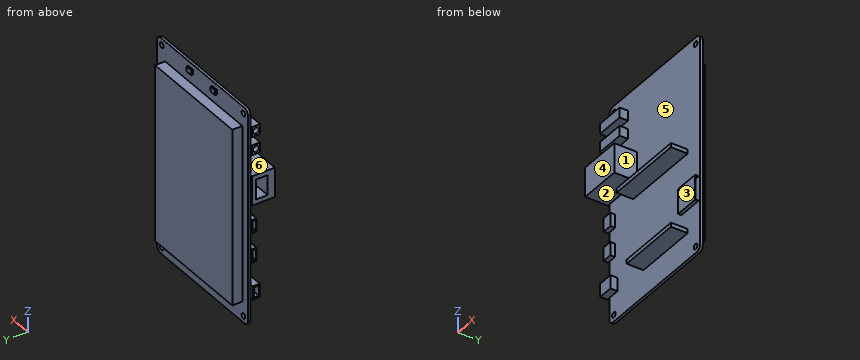
Autodesk Inventor part; units mm, degrees
ref_plane "YZ Plane" through (0, 0, 0) normal (1, 0, 0) x (0, 1, 0)
ref_plane "XZ Plane" through (0, 0, 0) normal (0, 1, 0) x (-1, 0, 0)
ref_plane "XY Plane" through (0, 0, 0) normal (0, 0, 1) x (1, 0, 0)
sketch "Esquisse1" plane through (0, 0, 0) normal (0, 1, 0) x (-1, 0, 0)
  line L0 (40, 65) -> (-40, 65)
  line L1 (-40, 65) -> (-40, -65)
  line L2 (-40, -65) -> (40, -65)
  line L3 (40, -65) -> (40, 65)
  point P0 (0, 0)
  dimension "d0" = 130
  dimension "d1" = 80
  dimension "d2" = 40
  dimension "d3" = 65
extrude "Extrusion1" add sketch "Esquisse1" along normal blind 1.6
sketch "Esquisse2" plane through (0, 1.6, 0) normal (0, 1, 0) x (1, 0, 0)
  circle A0 centre (-36, -61) radius 1.6
  circle A1 centre (-36, 61) radius 1.6
  circle A2 centre (36, 61) radius 1.6
  circle A3 centre (36, -61) radius 1.6
  point P0 (0, 0)
  dimension "d6" = 3.2
  dimension "d7" = 3.2
  dimension "d8" = 3.2
  dimension "d9" = 3.2
  dimension "d10" = 122
  dimension "d11" = 122
  dimension "d12" = 72
  dimension "d13" = 72
  dimension "d14" = 61
  dimension "d15" = 36
  dimension "d16" = 36
  dimension "d17" = 61
extrude "Extrusion2" cut sketch "Esquisse2" against normal blind 1.6
fillet "Congé1" radius 3.2 4 edges at (-40, 0.8, 65) (40, 0.8, 65) (40, 0.8, -65) (-40, 0.8, -65)
sketch "Esquisse3" plane through (0, 1.6, 0) normal (0, 1, 0) x (1, 0, 0)
  line L0 (-35, -53) -> (33, -53)
  line L1 (33, -53) -> (33, 53)
  line L2 (33, 53) -> (-35, 53)
  line L3 (-35, 53) -> (-35, -53)
  line L4 (40, -61.8) -> (40, 61.8)
  line L5 (36.8, 65) -> (-36.8, 65)
  point P0 (0, 0)
  dimension "d21" = 106
  dimension "d22" = 68
  dimension "d23" = 7
  dimension "d24" = 12
extrude "Extrusion3" add sketch "Esquisse3" along normal blind 6
sketch "Esquisse4" plane through (0, 1.6, 0) normal (0, 1, 0) x (1, 0, 0)
  line L0 (-12.5, -59) -> (-8.5, -59)
  line L1 (-8.5, -59) -> (-8.5, -62)
  line L2 (-8.5, -62) -> (-12.5, -62)
  line L3 (-12.5, -62) -> (-12.5, -59)
  line L4 (8.5, -59) -> (12.5, -59)
  line L5 (12.5, -59) -> (12.5, -62)
  line L6 (12.5, -62) -> (8.5, -62)
  line L7 (8.5, -62) -> (8.5, -59)
  line L8 (-36.8, -65) -> (36.8, -65)
  line L9 (40, -61.8) -> (40, 61.8)
  point P0 (0, 0)
  dimension "d27" = 4
  dimension "d28" = 3
  dimension "d29" = 6
  dimension "d30" = 6
  dimension "d31" = 4
  dimension "d32" = 17
  dimension "d33" = 27.5
extrude "Extrusion4" add sketch "Esquisse4" along normal blind 1
sketch "Esquisse5" plane through (0, 0, 0) normal (0, -1, 0) x (1, 0, 0)
  line L0 (-41.9, -48.5) -> (-32.9, -48.5)
  line L1 (-32.9, -48.5) -> (-32.9, -40.5)
  line L2 (-32.9, -40.5) -> (-41.9, -40.5)
  line L3 (-41.9, -40.5) -> (-41.9, -48.5)
  line L4 (36.8, -65) -> (-36.8, -65)
  line L5 (-40, -61.8) -> (-40, 61.8)
  point P0 (0, 0)
  dimension "d36" = 8
  dimension "d37" = 9
  dimension "d38" = 16.5
  dimension "d39" = 1.9
extrude "Extrusion5" add sketch "Esquisse5" along normal blind 4.2
sketch "Esquisse6" plane through (0, 0, 0) normal (0, -1, 0) x (1, 0, 0)
  line L0 (-35, 53) -> (-35, -53)
  line L1 (-41, -26.7) -> (-35, -26.7)
  line L2 (-35, -26.7) -> (-35, -18.7)
  line L3 (-35, -18.7) -> (-41, -18.7)
  line L4 (-41, -18.7) -> (-41, -26.7)
  line L5 (-41, -9.1) -> (-35, -9.1)
  line L6 (-35, -9.1) -> (-35, -1.1)
  line L7 (-35, -1.1) -> (-41, -1.1)
  line L8 (-41, -1.1) -> (-41, -9.1)
  line L9 (-32.9, -40.5) -> (-41.9, -40.5)
  line L10 (-40, -61.8) -> (-40, 61.8)
  point P0 (0, 0)
  dimension "d42" = 8
  dimension "d43" = 8
  dimension "d44" = 6
  dimension "d45" = 13.8
  dimension "d46" = 9.6
  dimension "d47" = 1
extrude "Extrusion6" add sketch "Esquisse6" along normal blind 2.8 contours L0 L5 L10 L7 | L10 L5 L8 L7 | L0 L1 L10 L3 | L10 L1 L4 L3
sketch "Esquisse7" plane through (0, 0, 0) normal (0, -1, 0) x (1, 0, 0)
  line L0 (-41.4, 7.9) -> (-15.7, 7.9)
  line L1 (-15.7, 7.9) -> (-15.7, 25.6)
  line L2 (-15.7, 25.6) -> (-41.4, 25.6)
  line L3 (-41.4, 25.6) -> (-41.4, 7.9)
  line L4 (-35, -1.1) -> (-41, -1.1)
  line L5 (-40, -1.1) -> (-40, 61.8)
  point P0 (0, 0)
  dimension "d50" = 25.7
  dimension "d51" = 17.7
  dimension "d52" = 9
  dimension "d53" = 1.4
extrude "Extrusion7" add sketch "Esquisse7" along normal blind 13.6
sketch "Esquisse8" plane through (0, 0, 0) normal (0, -1, 0) x (1, 0, 0)
  line L0 (-41, 38) -> (-23.6, 38)
  line L1 (-23.6, 38) -> (-23.6, 44)
  line L2 (-23.6, 44) -> (-41, 44)
  line L3 (-41, 44) -> (-41, 38)
  line L4 (-41, 49) -> (-23.6, 49)
  line L5 (-23.6, 49) -> (-23.6, 55)
  line L6 (-23.6, 55) -> (-41, 55)
  line L7 (-41, 55) -> (-41, 49)
  line L8 (-15.7, 25.6) -> (-41.4, 25.6)
  line L9 (-40, 25.6) -> (-40, 61.8)
  point P0 (0, 0)
  dimension "d56" = 6
  dimension "d57" = 6
  dimension "d58" = 17.4
  dimension "d59" = 5
  dimension "d60" = 12.4
  dimension "d61" = 1
extrude "Extrusion8" add sketch "Esquisse8" along normal blind 5
sketch "Esquisse9" plane through (-41.4, 0, 7.9) normal (-1, 0, 0) x (0, 0, 1)
  line L0 (2.85, -2.2) -> (14.85, -2.2)
  line L1 (14.85, -2.2) -> (14.85, -9.2)
  line L2 (14.85, -9.2) -> (2.85, -9.2)
  line L3 (2.85, -9.2) -> (2.85, -2.2)
  line L4 (17.7, 0) -> (0, 0)
  line L5 (17.7, 0) -> (17.7, -13.6)
  line L6 (0, 0) -> (0, -13.6)
  point P0 (-7.9, 0)
  dimension "d64" = 12
  dimension "d65" = 7
  dimension "d66" = 2.2
  dimension "d67" = 17.7
  dimension "d68" = 2.85
extrude "Extrusion9" cut sketch "Esquisse9" against normal blind 11
sketch "Esquisse10" plane through (-41.9, 0, -48.5) normal (-1, 0, 0) x (0, 0, 1)
  line L0 (1, -0.6) -> (7, -0.6)
  line L1 (7, -0.6) -> (7, -3.6)
  line L2 (7, -3.6) -> (1, -3.6)
  line L3 (1, -3.6) -> (1, -0.6)
  line L4 (22.55, -0.4) -> (29.05, -0.4)
  line L5 (29.05, -0.4) -> (29.05, -2.4)
  line L6 (29.05, -2.4) -> (22.55, -2.4)
  line L7 (22.55, -2.4) -> (22.55, -0.4)
  line L8 (40.15, -0.4) -> (46.65, -0.4)
  line L9 (46.65, -0.4) -> (46.65, -2.4)
  line L10 (46.65, -2.4) -> (40.15, -2.4)
  line L11 (40.15, -2.4) -> (40.15, -0.4)
  circle A0 centre (89.5, -2.5) radius 1.8
  circle A1 centre (100.5, -2.5) radius 1.8
  line L12 (8, 0) -> (0, 0)
  line L13 (8, -4.2) -> (0, -4.2)
  line L14 (8, 0) -> (8, -4.2)
  line L15 (0, 0) -> (0, -4.2)
  line L16 (29.8, 0) -> (21.8, 0)
  line L17 (29.8, -2.8) -> (21.8, -2.8)
  line L18 (29.8, 0) -> (29.8, -2.8)
  line L19 (21.8, 0) -> (21.8, -2.8)
  line L20 (47.4, 0) -> (47.4, -2.8)
  line L21 (39.4, 0) -> (39.4, -2.8)
  line L22 (92.5, 0) -> (92.5, -5)
  line L23 (86.5, 0) -> (86.5, -5)
  line L24 (92.5, 0) -> (86.5, 0)
  line L25 (92.5, -5) -> (86.5, -5)
  line L26 (97.5, 0) -> (97.5, -5)
  point P0 (48.5, 0)
  dimension "d71" = 3
  dimension "d72" = 2
  dimension "d73" = 2
  dimension "d74" = 6
  dimension "d75" = 6.5
  dimension "d76" = 6.5
  dimension "d77" = 4.2
  dimension "d78" = 8
  dimension "d79" = 2.8
  dimension "d80" = 8
  dimension "d81" = 8
  dimension "d82" = 1
  dimension "d83" = 0.6
  dimension "d84" = 0.75
  dimension "d86" = 0.4
  dimension "d87" = 0.75
  dimension "d88" = 6
  dimension "d89" = 5
  dimension "d90" = 3
  dimension "d91" = 2.5
  dimension "d92" = 3
  dimension "d93" = 2.5
  dimension "d94" = 3.6
  dimension "d95" = 3.6
extrude "Extrusion10" cut sketch "Esquisse10" against normal blind 4 contours L0 L1 L2 L3 | L4 L5 L6 L7 | L8 L9 L10 L11 | A0 | A1
sketch "Esquisse11" plane through (0, 0, 0) normal (0, -1, 0) x (1, 0, 0)
  line L0 (38.5, -35) -> (23.5, -35)
  line L1 (23.5, -35) -> (23.5, -20)
  line L2 (23.5, -20) -> (38.5, -20)
  line L3 (38.5, -20) -> (38.5, -35)
  line L4 (40, 61.8) -> (40, -61.8)
  line L5 (36.8, -65) -> (-36.8, -65)
  point P0 (0, 0)
  dimension "d98" = 15
  dimension "d99" = 15
  dimension "d100" = 1.5
  dimension "d101" = 30
extrude "Extrusion11" add sketch "Esquisse11" along normal blind 2
sketch "Esquisse13" plane through (38.5, 0, -20) normal (1, 0, 0) x (0, 0, -1)
  line L0 (-1.3, 0) -> (6.7, 0)
  line L1 (14.7, -1.7) -> (0.3, -1.7)
  line L2 (0.3, -1.7) -> (0.3, 0)
  line L3 (0.3, 0) -> (14.7, 0)
  line L4 (14.7, 0) -> (14.7, -1.7)
  line L5 (0, 0) -> (0, -2)
  line L6 (15, 0) -> (15, -2)
  point P0 (-20, 0)
  dimension "d104" = 0.3
  dimension "d106" = 0.3
  dimension "d107" = 0.3
extrude "Extrusion12" cut sketch "Esquisse13" against normal blind 12
sketch "Esquisse14" plane through (0, 0, 0) normal (0, -1, 0) x (1, 0, 0)
  line L0 (-10, -49) -> (29, -49)
  line L1 (29, -49) -> (29, -46.5)
  line L2 (29, -46.5) -> (-10, -46.5)
  line L3 (-10, -46.5) -> (-10, -49)
  line L4 (-19, -1) -> (29, -1)
  line L5 (29, -1) -> (29, 1.5)
  line L6 (29, 1.5) -> (-19, 1.5)
  line L7 (-19, 1.5) -> (-19, -1)
  line L8 (40, 61.8) -> (40, -61.8)
  line L9 (36.8, -65) -> (-36.8, -65)
  point P0 (0, 0)
  dimension "d110" = 2.5
  dimension "d111" = 2.5
  dimension "d112" = 39
  dimension "d113" = 48
  dimension "d114" = 11
  dimension "d115" = 16
  dimension "d116" = 64
extrude "Extrusion13" add sketch "Esquisse14" along normal blind 10
equation "\"d31\" = d27"
equation "\"d43\" = d42"
equation "\"d57\" = d56"
equation "\"d68\" = -0.5 * d64 + 0.5 * d67"
equation "\"d82\" = -0.5 * d74 + 0.5 * d78"
equation "\"d83\" = -0.5 * d71 + 0.5 * d77"
equation "\"d84\" = -0.5 * d75 + 0.5 * d80"
equation "\"d86\" = -0.5 * d72 + 0.5 * d79"
equation "\"d87\" = -0.5 * d76 + 0.5 * d81"
equation "\"d90\" = 0.5 * d88"
equation "\"d91\" = 0.5 * d89"
equation "\"d92\" = d90"
equation "\"d93\" = d91"
equation "\"d95\" = d94"
equation "\"d106\" = d104"
equation "\"d107\" = d104"
equation "\"d111\" = d110"
properties part number "STM32F746G-Disco"
The model under review builds one solid part; all positions refer to its coordinate system, in mm. Face numbers are marked on the shaded views. A direction names the side the tool comes from. Give positions to 0.01 mm unless a question says otherwise; leave off trailing zeros. Write each loop counter-clockwise with the first axis right and the second up, starting at its lowest first coordinate (ties: lowest second). Pieces come first, ordered by that corner, then holes.
1. Draft analysis for pull direction Z (two halves, no side actions). For the marked faces 4, 5 and 6, state which applies: +Z half, -Z half, draft (parallel to the pull), parting line (faces both ways), or undercut.
2. Wall thickness on L1, parallel to X at y = 0.55, z = 61; L2, parallel to Z at x = 36, y = 1; L3, parallel to Y at x = -40.1, z = 41: over which ranges is each line inside the solid? List them lowest first.
3. Add section C-C, the plane y = -11.75. Write out the cut boundary in (x, z), plus the area to 3 significant figures.
4. For P1, Ø3, axis at x = 2.5, z = 0.5, coming from the -Y side; P2, Ø8, axis at x = -2, y = -5, coming from the -Z side; P3, Ø7, axis at y = -5, z = 20, coming from the +X side; P4, Ø3, axis at x = 36, z = -61, coming from the -Y side, all flat-tipped, find the tip position at first contact; note any pin that passes through.
5. Add section B-B, the plane x = 0. Write out the cut boundary in (y, z).
6. Add section A-A, the plane z = 31. Write out the cut boundary in (x, y).
7. Add section D-D, the plane z = -56.5. Write out the cut boundary in (x, y), plus the area to 3 significant figures.
8. Tool access review of the marked faces 1, 2 and 3: name each direction out of +Z, -Z, +X, -X, +Y, -Y from which nothing blocks a thin tool from reaching the whole face with its end or side.
Worked answers:
1. face 4: draft
1. face 5: undercut
1. face 6: undercut
2. L1: x = -40 to -37.6, -34.4 to 34.4, 37.6 to 40
2. L2: z = -65 to -62.6, -59.4 to 59.4, 62.6 to 65
2. L3: y = -5 to -4.3, -0.7 to 0
3. outline: (-41.4, 7.9) - (-15.7, 7.9) - (-15.7, 25.6) - (-41.4, 25.6) - close
3. area: 455 mm2
4. P1: stops at y = -10
4. P2: stops at z = -49
4. P3: stops at x = -15.7
4. P4: passes through
5. outline: (-10, -49) - (0, -49) - (0, -65) - (1.6, -65) - (1.6, -53) - (7.6, -53) - (7.6, 53) - (1.6, 53) - (1.6, 65) - (0, 65) - (0, 1.5) - (-10, 1.5) - (-10, -1) - (0, -1) - (0, -46.5) - (-10, -46.5) - close
6. outline: (-40, 0) - (40, 0) - (40, 1.6) - (33, 1.6) - (33, 7.6) - (-35, 7.6) - (-35, 1.6) - (-40, 1.6) - close
7. outline: (-40, 0) - (40, 0) - (40, 1.6) - (-40, 1.6) - close
7. area: 128 mm2
8. face 1: +Z, +X, -Y
8. face 2: +X, -X, -Y
8. face 3: +X, -Y
